Part model, mm, in its own coordinate system. Face numbers are marked on the shaded views. A direction names the side the tool comes from. Round coordinates to 2 decimals unless told otherwise and drop trailing zeros. Loops run counter-clockwise (first coordinate to the right, second up) from the corner with the lowest first, then second, coordinate; pieces in that order, holes last. Notation, with made-up numbers: M 11.25,67.25 L 27.25,67.25 A22 cw 27.25,84.25 Z; hole C 47,4.25 d9. An arc over 180 degrees is marked long. Put each result on its own line as item: value. Start each with the question number.
1) Slice it at B-B on x = 41.5. Give the cut face in (y, z), then the cut area to 3 significant figures.
2) Which spindle directions (+Z, -Z, +X, -X, +Y, -Y) get a long thin tool onto all of the face, cutting with end or side? Do the marked faces 1 and 2. Say none if no direction does.
3) Probe line 1 along Y through (x, z) = (22.5, 24); line 2 along Z through (x, y) = (3.5, 2.5); line 3 along Y through (x, z) = (-8, 12). List the from-to ranges inside material, lowest first.
4) Slice it at C-C on y = 61.5. Give the cut face in (x, z), then the cut area to 3 significant figures.
5) Slice it at A-A on y = 23.5. Give the cut face in (x, z).
6) Drop flat-ended pins along their axis: pin 1 Ø1 at (x, z) = (12.5, 22.5) entering from +Y; pin 2 Ø23 at (x, z) = (-14.5, 17.5) entering from +Y; pin 3 Ø1 at (x, z) = (31.5, 11.5) entering from +Y. Give the stop position or say it passes through.
7) Pull direction Z, two halves, no side cores. Call the marked faces 3, 4 and 5: +Z half, -Z half, draft (parallel to the pull), parting line (faces both ways), or undercut.
Autodesk Inventor part; units mm, degrees
ref_plane "YZ Plane" through (0, 0, 0) normal (1, 0, 0) x (0, 1, 0)
ref_plane "XZ Plane" through (0, 0, 0) normal (0, 1, 0) x (-1, 0, 0)
ref_plane "XY Plane" through (0, 0, 0) normal (0, 0, 1) x (1, 0, 0)
sketch "Sketch1" plane through (0, 0, 0) normal (0, 1, 0) x (-1, 0, 0)
  circle A0 centre (0, 0) radius 5.95
  circle A1 centre (0, 0) radius 8
  circle A2 centre (0, 0) radius 30
  dimension "d0" = 11.9
  dimension "d2" = 16
  dimension "d3" = 60
extrude "Extrusion1" add sketch "Sketch1" along normal blind 70 contours A0
extrude "Extrusion2" cut sketch "Sketch1" along normal blind 45 contours A1
extrude "Extrusion3" add sketch "Sketch1" along normal blind 45 contours A0 | A1
extrude "Extrusion4" add sketch "Sketch1" along normal blind 12 contours A2
sketch "Sketch2" plane through (0, 0, 0) normal (0, -1, 0) x (1, 0, 0)
  line L0 (-50, 38) -> (50, 38)
  line L1 (50, 38) -> (50, -38)
  line L2 (50, -38) -> (-50, -38)
  line L3 (-50, -38) -> (-50, 38)
  line L4 (-50, 38) -> (50, -38) construction
  line L5 (50, 38) -> (-50, -38) construction
  point P0 (0, 0)
  dimension "d12" = 100
extrude "Extrusion5" add sketch "Sketch2" along normal blind 2
fillet "Fillet1" radius 16 4 edges at (50, -1, 38) (50, -1, -38) (-50, -1, -38) (-50, -1, 38)
fillet "Fillet2" radius 16 1 edges at (30, 12, 0)
sketch "Sketch3" plane through (34, 0, -38) normal (0, 0, -1) x (-1, 0, 0)
  line L0 (0, 0) -> (68, 0)
  line L1 (0, -2) -> (68, -2)
  line L2 (68, -2) -> (68, 0)
  line L3 (68, 0) -> (0, 0)
  line L4 (0, 0) -> (0, -2)
  point P0 (34, 0)
extrude "Extrusion6" add sketch "Sketch3" along normal blind 4
sketch "Sketch4" plane through (0, 0, 0) normal (0, 1, 0) x (1, 0, 0)
  line L0 (-34, 42) -> (34, 42)
  line L1 (-34, 38) -> (-34, 42)
  line L2 (34, 42) -> (-34, 42)
  line L3 (-34, 42) -> (-34, 38)
  line L4 (-34, 38) -> (34, 38)
  line L5 (34, 38) -> (34, 42)
  point P0 (0, 0)
extrude "Extrusion7" add sketch "Sketch4" along normal blind 5
fillet "Fillet3" radius 3 3 edges at (0, 5, -42) (-34, 1.5, -42) (34, 1.5, -42)
fillet "Fillet4" radius 1 1 edges at (0, 5, -38)
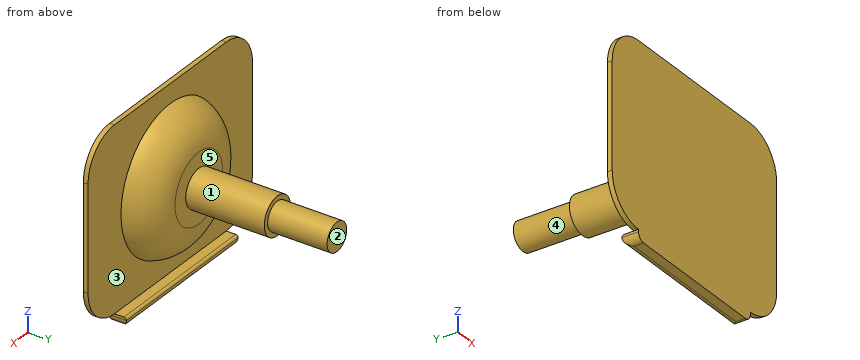
Recorded:
1. outline: M -2,-36.13 L 0,-36.13 L 0,36.13 L -2,36.13 Z
1. area: 145 mm2
2. face 1: +Y
2. face 2: +Z, -Z, +X, -X, +Y
3. line 1: y = -2 to 0
3. line 2: z = -41.96 to -38, -28.92 to 28.92
3. line 3: y = -2 to 12
4. outline: C 0,0 d11.9
4. area: 111 mm2
5. outline: C 0,0 d16
6. pin 1: stops at y = 7.87
6. pin 2: stops at y = 12
6. pin 3: stops at y = 0
7. face 3: undercut
7. face 4: parting line
7. face 5: draft
